from build123d import *

# Parameters (mm, degrees)
SKETCH_1_R      = 5
SKETCH_1_R_2    = 1.5
SKETCH_1_R_3    = 8
SKETCH_1_R_4    = 2.5
EXTRUDE_1_DEPTH = 5


with BuildPart() as part:
    # 草图1 → 凸台-拉伸1 (new body)
    with BuildSketch(Plane.XY):
        with BuildLine():
            Line((-26, 220), (-26, 0))
            ThreePointArc((-26, 0), (0, -26), (26, 0))
            Line((26, 0), (26, 220))
            ThreePointArc((26, 220), (0, 246), (-26, 220))
        make_face()
        Circle(SKETCH_1_R, mode=Mode.SUBTRACT)
        with Locations((0, -14)):
            Circle(SKETCH_1_R_2, mode=Mode.SUBTRACT)
        with Locations(Location((0, 220, 0), (0, 0, 180))):
            Circle(SKETCH_1_R_3, mode=Mode.SUBTRACT)
        with Locations((-14, 0)):
            Circle(SKETCH_1_R_2, mode=Mode.SUBTRACT)
        with Locations((0, 14)):
            Circle(SKETCH_1_R_2, mode=Mode.SUBTRACT)
        with Locations((14, 0)):
            Circle(SKETCH_1_R_2, mode=Mode.SUBTRACT)
        with Locations((-21, 62)):
            Circle(SKETCH_1_R_4, mode=Mode.SUBTRACT)
        with Locations((21, 62)):
            Circle(SKETCH_1_R_4, mode=Mode.SUBTRACT)
        with Locations((0, 234)):
            Circle(SKETCH_1_R_2, mode=Mode.SUBTRACT)
        with Locations((14, 220)):
            Circle(SKETCH_1_R_2, mode=Mode.SUBTRACT)
        with Locations((0, 206)):
            Circle(SKETCH_1_R_2, mode=Mode.SUBTRACT)
        with Locations((-14, 220)):
            Circle(SKETCH_1_R_2, mode=Mode.SUBTRACT)
        with BuildLine():
            Line((-3, 23), (-3, 53))
            ThreePointArc((-3, 53), (0, 56), (3, 53))
            Line((3, 53), (3, 23))
            ThreePointArc((3, 23), (0, 20), (-3, 23))
        make_face(mode=Mode.SUBTRACT)
        with BuildLine():
            Line((-17, 23), (-17, 53))
            ThreePointArc((-17, 53), (-14, 56), (-11, 53))
            Line((-11, 53), (-11, 23))
            ThreePointArc((-11, 23), (-14, 20), (-17, 23))
        make_face(mode=Mode.SUBTRACT)
        with BuildLine():
            Line((17, 23), (17, 53))
            ThreePointArc((17, 53), (14, 56), (11, 53))
            Line((11, 53), (11, 23))
            ThreePointArc((11, 23), (14, 20), (17, 23))
        make_face(mode=Mode.SUBTRACT)
        with BuildLine():
            Line((-3, 105.5), (-3, 135.5))
            ThreePointArc((-3, 135.5), (0, 138.5), (3, 135.5))
            Line((3, 135.5), (3, 105.5))
            ThreePointArc((3, 105.5), (0, 102.5), (-3, 105.5))
        make_face(mode=Mode.SUBTRACT)
        with BuildLine():
            Line((-17, 105.5), (-17, 135.5))
            ThreePointArc((-17, 135.5), (-14, 138.5), (-11, 135.5))
            Line((-11, 135.5), (-11, 105.5))
            ThreePointArc((-11, 105.5), (-14, 102.5), (-17, 105.5))
        make_face(mode=Mode.SUBTRACT)
        with BuildLine():
            Line((17, 105.5), (17, 135.5))
            ThreePointArc((17, 135.5), (14, 138.5), (11, 135.5))
            Line((11, 135.5), (11, 105.5))
            ThreePointArc((11, 105.5), (14, 102.5), (17, 105.5))
        make_face(mode=Mode.SUBTRACT)
    extrude(amount=EXTRUDE_1_DEPTH)


solid = part.part
Read the model definition and answer for the solid it produces. Units are mm, in the model's axes. A direction names the side the tool comes from. Coordinates: 2 decimals unless noted, no trailing zeros. Write each loop counter-clockwise with the first axis right and the second up, starting at its lowest first coordinate (ties: lowest second). Pieces come first, ordered by that corner, then holes. Notation, with made-up numbers: M -37,-26.75 L -17,-26.75 A19 cw -17,3.25 Z; hole C 54.5,-31.75 d4. An arc over 180 degrees is marked long. Use a Markdown table: item, result.
Q1. The part is cut by section B-B, the plane z = 4. Give the number of separate pieces and of enclosed holes in the cut face, then the cut area to 3 significant figures.
Answer block:
| item | result |
|---|---|
| separate pieces | 1 |
| enclosed holes | 18 |
| area | 11,900 mm2 |
Q2. Each of these flat-tipped pins is pushed along its axis until it touches: pin 1 Ø4.5 at (x, y) = (-21, 62) entering from -Z; pin 2 Ø3 at (x, z) = (19, 4) entering from -Y; pin 3 Ø1 at (x, z) = (8.5, 4) entering from +Y. Where does it stop, or does it pass through?
Answer block:
| item | result |
|---|---|
| pin 1 | passes through |
| pin 2 | stops at y = -19.23 |
| pin 3 | stops at y = 244.74 |
Q3. Straight lines are drawn through the part: L1, parallel to X at y = 113.5, z = 3.8; L2, parallel to X at y = 220, z = 1.2; L3, parallel to X at y = 206, z = 3.8. For each, find the intervals that lie inside material, in ascending order. Write a range as [from, to].
Answer block:
| item | result |
|---|---|
| L1 | x = [-26, -17], [-11, -3], [3, 11], [17, 26] |
| L2 | x = [-26, -15.5], [-12.5, -8], [8, 12.5], [15.5, 26] |
| L3 | x = [-26, -1.5], [1.5, 26] |
Q4. The part is cut by section A-A, the plane x = -21. Write down the section's boundary in (y, z).
Answer block:
| item | result |
|---|---|
| outline | M -15.33,0 L 59.5,0 L 59.5,5 L -15.33,5 Z; M 64.5,0 L 235.33,0 L 235.33,5 L 64.5,5 Z |
Q5. Determine the mould class of faces 1 (the face through (-6, 112, 0)), 2 (the face through (-11, 38, 2)), 3 (the face through (-14.1, 138.5, 2.5)), 4 (the face through (-0.572, -25.994, 2.465)) for opening direction X: released by +X, released by -X, zero draft, split by the parting line, or undercut.
Answer block:
| item | result |
|---|---|
| face 1 | zero draft |
| face 2 | undercut |
| face 3 | undercut |
| face 4 | split by the parting line |
Q6. Which of the six approach directions +Z, -Z, +X, -X, +Y, -Y give full straight-line access (tool end or side, diameter ignored) to faces 5 (the face through (-14, 20, 2)), 6 (the face through (26, 108, 2))?
Answer block:
| item | result |
|---|---|
| face 5 | +Z, -Z |
| face 6 | +Z, -Z, +X, +Y, -Y |
